Source: CAD feature listing. Evaluate the final solid. Frame: model axes, mm. Give positions to 0.01 mm unless a question says otherwise; leave off trailing zeros.
from build123d import *

# Parameters (mm, degrees)
MODEL_W                 = 3
MODEL_H                 = 3
SALIENTE_EXTRUIR1_DEPTH = 3


with BuildPart() as part:
    # Model → Saliente-Extruir1 (new body)
    with BuildSketch(Plane.XY):
        with BuildLine():
            Line((139.892723231, 274.571078663), (139.892723231, 292.568350817))
            ThreePointArc((139.892723231, 292.568350817), (138.574703747, 295.750331332), (135.392723231, 297.068350817))
            Line((135.392723231, 297.068350817), (9.392723231, 297.068350817))
            ThreePointArc((9.392723231, 297.068350817), (6.210742716, 295.750331332), (4.892723231, 292.568350817))
            Line((4.892723231, 292.568350817), (4.892723231, 274.571078663))
            ThreePointArc((4.892723231, 274.571078663), (6.210742716, 271.389098148), (9.392723231, 270.071078663))
            Line((9.392723231, 270.071078663), (135.392723231, 270.071078663))
            ThreePointArc((135.392723231, 270.071078663), (138.574703747, 271.389098148), (139.892723231, 274.571078663))
        make_face()
        with Locations((9.392723231, 292.568350816)):
            Rectangle(MODEL_W, MODEL_H, mode=Mode.SUBTRACT)
        with Locations((18.392723231, 292.568350816)):
            Rectangle(MODEL_W, MODEL_H, mode=Mode.SUBTRACT)
        with Locations((27.392723231, 292.568350816)):
            Rectangle(MODEL_W, MODEL_H, mode=Mode.SUBTRACT)
        with Locations((36.392723231, 292.568350816)):
            Rectangle(MODEL_W, MODEL_H, mode=Mode.SUBTRACT)
        with Locations((45.392723231, 292.568350816)):
            Rectangle(MODEL_W, MODEL_H, mode=Mode.SUBTRACT)
        with Locations((54.392723231, 292.568350816)):
            Rectangle(MODEL_W, MODEL_H, mode=Mode.SUBTRACT)
        with Locations((63.392723231, 292.568350816)):
            Rectangle(MODEL_W, MODEL_H, mode=Mode.SUBTRACT)
        with Locations((72.392723231, 292.568350816)):
            Rectangle(MODEL_W, MODEL_H, mode=Mode.SUBTRACT)
        with Locations((81.392723231, 292.568350816)):
            Rectangle(MODEL_W, MODEL_H, mode=Mode.SUBTRACT)
        with Locations((90.392723231, 292.568350816)):
            Rectangle(MODEL_W, MODEL_H, mode=Mode.SUBTRACT)
        with Locations((99.392723231, 292.568350816)):
            Rectangle(MODEL_W, MODEL_H, mode=Mode.SUBTRACT)
        with Locations((108.392723231, 292.568350816)):
            Rectangle(MODEL_W, MODEL_H, mode=Mode.SUBTRACT)
        with Locations((117.392723231, 292.568350816)):
            Rectangle(MODEL_W, MODEL_H, mode=Mode.SUBTRACT)
        with Locations((126.392723231, 292.568350816)):
            Rectangle(MODEL_W, MODEL_H, mode=Mode.SUBTRACT)
        with Locations((135.392723231, 292.568350816)):
            Rectangle(MODEL_W, MODEL_H, mode=Mode.SUBTRACT)
        with Locations((9.392723231, 283.568350816)):
            Rectangle(MODEL_W, MODEL_H, mode=Mode.SUBTRACT)
        with Locations((18.392723231, 283.568350816)):
            Rectangle(MODEL_W, MODEL_H, mode=Mode.SUBTRACT)
        with Locations((27.392723231, 283.568350816)):
            Rectangle(MODEL_W, MODEL_H, mode=Mode.SUBTRACT)
        with Locations((36.392723231, 283.568350816)):
            Rectangle(MODEL_W, MODEL_H, mode=Mode.SUBTRACT)
        with Locations((45.392723231, 283.568350816)):
            Rectangle(MODEL_W, MODEL_H, mode=Mode.SUBTRACT)
        with Locations((54.392723231, 283.568350816)):
            Rectangle(MODEL_W, MODEL_H, mode=Mode.SUBTRACT)
        with Locations((63.392723231, 283.568350816)):
            Rectangle(MODEL_W, MODEL_H, mode=Mode.SUBTRACT)
        with Locations((72.392723231, 283.568350816)):
            Rectangle(MODEL_W, MODEL_H, mode=Mode.SUBTRACT)
        with Locations((81.392723231, 283.568350816)):
            Rectangle(MODEL_W, MODEL_H, mode=Mode.SUBTRACT)
        with Locations((90.392723231, 283.568350816)):
            Rectangle(MODEL_W, MODEL_H, mode=Mode.SUBTRACT)
        with Locations((99.392723231, 283.568350816)):
            Rectangle(MODEL_W, MODEL_H, mode=Mode.SUBTRACT)
        with Locations((108.392723231, 283.568350816)):
            Rectangle(MODEL_W, MODEL_H, mode=Mode.SUBTRACT)
        with Locations((117.392723231, 283.568350816)):
            Rectangle(MODEL_W, MODEL_H, mode=Mode.SUBTRACT)
        with Locations((126.392723231, 283.568350816)):
            Rectangle(MODEL_W, MODEL_H, mode=Mode.SUBTRACT)
        with Locations((135.392723231, 283.568350816)):
            Rectangle(MODEL_W, MODEL_H, mode=Mode.SUBTRACT)
        with Locations((9.392723231, 274.568350816)):
            Rectangle(MODEL_W, MODEL_H, mode=Mode.SUBTRACT)
        with Locations((18.392723231, 274.568350816)):
            Rectangle(MODEL_W, MODEL_H, mode=Mode.SUBTRACT)
        with Locations((27.392723231, 274.568350816)):
            Rectangle(MODEL_W, MODEL_H, mode=Mode.SUBTRACT)
        with Locations((36.392723231, 274.568350816)):
            Rectangle(MODEL_W, MODEL_H, mode=Mode.SUBTRACT)
        with Locations((45.392723231, 274.568350816)):
            Rectangle(MODEL_W, MODEL_H, mode=Mode.SUBTRACT)
        with Locations((54.392723231, 274.568350816)):
            Rectangle(MODEL_W, MODEL_H, mode=Mode.SUBTRACT)
        with Locations((63.392723231, 274.568350816)):
            Rectangle(MODEL_W, MODEL_H, mode=Mode.SUBTRACT)
        with Locations((72.392723231, 274.568350816)):
            Rectangle(MODEL_W, MODEL_H, mode=Mode.SUBTRACT)
        with Locations((81.392723231, 274.568350816)):
            Rectangle(MODEL_W, MODEL_H, mode=Mode.SUBTRACT)
        with Locations((90.392723231, 274.568350816)):
            Rectangle(MODEL_W, MODEL_H, mode=Mode.SUBTRACT)
        with Locations((99.392723231, 274.568350816)):
            Rectangle(MODEL_W, MODEL_H, mode=Mode.SUBTRACT)
        with Locations((108.392723231, 274.568350816)):
            Rectangle(MODEL_W, MODEL_H, mode=Mode.SUBTRACT)
        with Locations((117.392723231, 274.568350816)):
            Rectangle(MODEL_W, MODEL_H, mode=Mode.SUBTRACT)
        with Locations((126.392723231, 274.568350816)):
            Rectangle(MODEL_W, MODEL_H, mode=Mode.SUBTRACT)
        with Locations((135.392723231, 274.568350816)):
            Rectangle(MODEL_W, MODEL_H, mode=Mode.SUBTRACT)
    extrude(amount=SALIENTE_EXTRUIR1_DEPTH)


solid = part.part
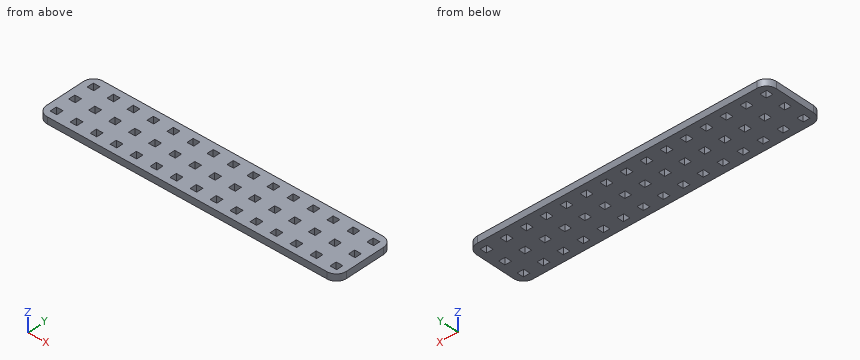
(1) Pin query (flat end, axial travel): pin 1 Ø8 at (x, y) = (85, 291) entering from -Z. Return the tip coordinate at first contact, or that it passes through.
(2) Line query: line 1 along Y through (x, z) = (71.5, 0.7); line 2 along X through (y, z) = (295.5, 2.15); line 3 along X through (y, z) = (271.5, 1.75). Output: solid intervals per line, ascending.
(3) Section A-A, the plane y = 283.75. Count the separate pieces of the cut face and the enclosed holes in it, plus the area to 3 significant figures.
Checks:
1. pin 1: stops at z = 0
2. line 1: y = 270.07 to 273.07, 276.07 to 282.07, 285.07 to 291.07, 294.07 to 297.07
2. line 2: x = 5.98 to 138.81
2. line 3: x = 6.1 to 138.68
3. separate pieces: 16
3. enclosed holes: 0
3. area: 270 mm2
